Autodesk Inventor part; units mm, degrees
ref_plane "YZ Plane" through (0, 0, 0) normal (1, 0, 0) x (0, 1, 0)
ref_plane "XZ Plane" through (0, 0, 0) normal (0, 1, 0) x (-1, 0, 0)
ref_plane "XY Plane" through (0, 0, 0) normal (0, 0, 1) x (1, 0, 0)
sketch "Sketch1" plane through (0, 0, 0) normal (0, 1, 0) x (-1, 0, 0)
  circle A0 centre (0, 0) radius 7
  circle A1 centre (0, 0) radius 9
  line L0 (7, 0) -> (9, 0)
  line L1 (9, 0) -> (8.6528, -2.4758)
  line L2 (9, 0) -> (8.6528, 2.4758)
  line L3 (8.6528, 2.4758) -> (0, 0)
  line L4 (0, 0) -> (8.6528, -2.4758)
  point P0 (6.7299, -1.9256)
  point P1 (6.7299, 1.9256)
  dimension "d0" = 14
  dimension "d1" = 18
  dimension "d2" = 2.5
  dimension "d3" = 2.5
extrude "Extrusion1" add sketch "Sketch1" along normal blind 6 contours A0 L4 A1 L3
fillet "Fillet1" radius 1 8 edges at (7, 0, 0) (9, 0, 0) (9, 6, 0) (7, 6, 0) (-8.6528, 3, -2.4758) (-6.7299, 3, -1.9256) (-8.6528, 3, 2.4758) (-6.7299, 3, 1.9256)
properties part number "CableRing"
Geometry: final body of the model. Coordinates: model frame, mm. Round coordinates to 2 decimals unless told otherwise and drop trailing zeros. Loops run counter-clockwise (first coordinate to the right, second up) from the corner with the lowest first, then second, coordinate; pieces in that order, holes last. Notation, with made-up numbers: (77, 65) -> (117, 65) arc R12 ccw to (117, 74) -> close; hole circle Ø5 at (85, 82.25). An arc over 180 degrees is marked (long way). Write each question's results on one line, items separated by ' | '.
Item 1: Line query: probe 1 along Z at (x, y) = (0, 4.25); probe 2 along X at (y, z) = (3, 0); probe 3 along Z at (x, y) = (4.25, 0.75). Output: solid intervals per line, ascending. Write a range as [from, to].
Answers below:
probe 1: z = [-9, -7], [7, 9] | probe 2: x = [7, 9] | probe 3: z = [-7.9, -5.6], [5.6, 7.9]
Item 2: Cut plane C-C on z = 0. Return the cut outline in (x, y), and give its area (3 significant figures).
Answers below:
outline: (7, 1) arc R1 ccw to (9, 1) -> (9, 5) arc R1 ccw to (7, 5) -> close | area: 11.1 mm²
Item 3: Cut plane B-B on y = 0.5. Return the cut outline in (x, z).
Answers below:
outline: (-8.34, -3) arc R8.87 ccw (long way) to (-8.34, 3) arc R1 ccw to (-6.73, 2.36) arc R7.13 cw (long way) to (-6.73, -2.36) arc R1 ccw to start
Item 4: Cut plane A-A on x = 0. Return the cut outline in (y, z).
Answers below:
outline: (1, -9) -> (5, -9) arc R1 ccw to (5, -7) -> (1, -7) arc R1 ccw to start; (1, 7) -> (5, 7) arc R1 ccw to (5, 9) -> (1, 9) arc R1 ccw to start
Item 5: Pin query (flat end, axial travel): pin 1 Ø3 at (y, z) = (5.5, -2) entering from -X; pin 2 Ø1.5 at (y, z) = (2.5, 5.5) entering from -X; pin 3 Ø10 at (x, z) = (-2, -1.5) entering from -Y. Return the tip coordinate at first contact, or that it passes through.
Answers below:
pin 1: stops at x = -8.36 | pin 2: stops at x = -7.64 | pin 3: stops at y = 0.13
Item 6: Pull-direction query (Z, two-part tool) for faces 1 (the face through (-7.729, 2.958, -2.217)), 2 (the face through (7, 3, 0)), 3 (the face through (9, 3, 0)); classes: pulls with the +Z half, pulls with the -Z half, needs draft (parallel to the pull), parting line crosses it, or undercut.
Answers below:
face 1: undercut | face 2: undercut | face 3: parting line crosses it
